from build123d import *

# Parameters (mm, degrees)
F0_W     = 215.9
F0_H     = 279.4
F1_DEPTH = 10.16
F3_DEPTH = 10.16
F4_W     = 25.4
F4_H     = 190.5
F5_DEPTH = 25.4
F6_R     = 6.35
F7_DEPTH = 25.4
F9_DEPTH = 25.4
F9_TAPER = 3


with BuildPart() as f1:
    # F0 (on Front) → F1 (new body)
    with BuildSketch(Plane.XZ):
        Rectangle(F0_W, F0_H)
    extrude(amount=F1_DEPTH)

    # F2 (on face) → F3 (join)
    with BuildSketch(Plane.XZ.offset(10.16)):
        Polygon((-56.5280616283, 184.6861541271), (-107.95, 139.7), (107.95, 139.7), (43.724745512, 184.6861541271), align=None)
    extrude(amount=-F3_DEPTH)

    # F4 (on face) → F5 (cut)
    with BuildSketch(Plane.XZ.offset(10.16)):
        with Locations((-76.9769162781, 0)):
            Rectangle(F4_W, F4_H)
        with Locations((76.6421729739, 0)):
            Rectangle(F4_W, F4_H)
    extrude(amount=-F5_DEPTH, mode=Mode.SUBTRACT)

    # F6 (on face) → F7 (cut)
    with BuildSketch(Plane.XZ.offset(10.16)):
        with Locations((-43.4066951275, 95.25)):
            Circle(F6_R)
        with Locations((-44.0643727779, 0)):
            Circle(F6_R)
        with Locations((-45.2269162781, -95.25)):
            Circle(F6_R)
        with Locations((46.7125048725, 95.25)):
            Circle(F6_R)
        with Locations((46.0548272221, 0)):
            Circle(F6_R)
        with Locations((44.8922837219, -95.25)):
            Circle(F6_R)
    extrude(amount=-F7_DEPTH, mode=Mode.SUBTRACT)

    # F8 (on face) → F9 (cut)
    with BuildSketch(Plane.XZ.offset(10.16)):
        with BuildLine():
            ThreePointArc((-64.2769162781, -139.7), (-57.5417241873, -136.9101920908), (-54.7519162781, -130.175))
            ThreePointArc((-54.7519162781, -130.175), (-71.0121083689, -123.4398079092), (-64.2769162781, -139.7))
        make_face()
        with BuildLine():
            ThreePointArc((73.4671729739, -130.175), (57.2069809313, -123.439807861), (63.9421728375, -139.7))
            ThreePointArc((63.9421728375, -139.7), (70.6773650165, -136.910192139), (73.4671729739, -130.175))
        make_face()
    extrude(amount=-F9_DEPTH, taper=F9_TAPER, mode=Mode.SUBTRACT)


solid = f1.part
CAD build for the part. Positions are in the model's coordinates, mm. A direction names the side the tool comes from. Give positions to 0.01 mm unless a question says otherwise; leave off trailing zeros. Loops run counter-clockwise (first coordinate to the right, second up) from the corner with the lowest first, then second, coordinate; pieces in that order, holes last. Notation, with made-up numbers: M -31,62 L 1,62 A22 cw 1,97 Z; hole C 76,-38 d2. An arc over 180 degrees is marked long. Answer in a Markdown table with one row per item. Add a question column.
Item 1: Mould opens along Z. For faces 1 (the face through (-107.95, -5, -2)), 2 (the face through (-6, -5, 184.686)), 3 (the face through (-66.28, -5.01, -139.21)) say: +Z half, -Z half, draft (parallel to the pull), parting line (faces both ways), or undercut.
Item 2: Drop flat-ended pins along their axis: P1, Ø5, axis at x = -81.5, y = -3.5, coming from the +Z side; P2, Ø3, axis at x = 81, y = -7.5, coming from the +Z side; P3, Ø11.5, axis at x = -45.23, z = -95.25, coming from the -Y side. Give the stop position or say it passes through.
Item 3: Band-saw the part on A-A on z = 0. Give the cut face in (x, y).
Item 4: Probe probe 1 along X at (y, z) = (-3.5, 14); probe 2 along X at (y, z) = (-0.75, 93); probe 3 along X at (y, z) = (-4, -124.5). List the from-to ranges inside material, lowest first.
Item 5: Band-saw the part on C-C on y = -2.75. Give the number of separate pieces and of enclosed holes in the cut face, then the cut area to 3 significant figures.
Item 6: Tool access for faces 4 (the face through (107.95, -5, -2)), 5 (the face through (76, -5, -95.25)): list every direction of +Z, -Z, +X, -X, +Y, -Y with a clear straight run to the whole face (end or side of a thin tool).
Item 7: Band-saw the part on B-B on x = 82.5. Give the cut face in (y, z), then the cut area to 3 significant figures.
Reply:
| question | item | result |
|---|---|---|
| 1 | face 1 | draft |
| 1 | face 2 | +Z half |
| 1 | face 3 | undercut |
| 2 | P1 | stops at z = 165.03 |
| 2 | P2 | stops at z = 159.63 |
| 2 | P3 | passes through |
| 3 | outline | M -107.95,-10.16 L -89.68,-10.16 L -89.68,0 L -107.95,0 Z; M -64.28,-10.16 L -50.41,-10.16 L -50.41,0 L -64.28,0 Z; M -37.71,-10.16 L 39.7,-10.16 L 39.7,0 L -37.71,0 Z; M 52.4,-10.16 L 63.94,-10.16 L 63.94,0 L 52.4,0 Z; M 89.34,-10.16 L 107.95,-10.16 L 107.95,0 L 89.34,0 Z |
| 4 | probe 1 | x = -107.95 to -89.68, -64.28 to 63.94, 89.34 to 107.95 |
| 4 | probe 2 | x = -107.95 to -89.68, -64.28 to -49.34, -37.47 to 40.77, 52.65 to 63.94, 89.34 to 107.95 |
| 4 | probe 3 | x = -107.95 to -71.52, -57.03 to 56.7, 71.19 to 107.95 |
| 5 | separate pieces | 1 |
| 5 | enclosed holes | 10 |
| 5 | area | 56,500 mm^2 |
| 6 | face 4 | +Z, -Z, +X, +Y, -Y |
| 6 | face 5 | +Y, -Y |
| 7 | outline | M -10.16,-139.7 L 0,-139.7 L 0,-95.25 L -10.16,-95.25 Z; M -10.16,95.25 L 0,95.25 L 0,157.53 L -10.16,157.53 Z |
| 7 | area | 1,080 mm^2 |
